Check sheet for the modelled part. Datum: model origin and axes. Units: mm. Coordinates: 2 decimals unless noted, no trailing zeros. Order: outer loops, then holes, each group sorted by start corner. A loop starts at its lowest first (then second) coordinate and runs counter-clockwise, first axis right, second up.
1. Cross-section at D-D (y = -14.5). Enter the section's corners in (x, z).
2. Draft check along Y on faces 1 (the cylindrical face through (4.68, 3.73, 0.99)), 2 (the flat face through (-20, -25.247, 1)), 3 (the flat face through (-11, -11, 0)). Enter one of: released by +Y, released by -Y, zero draft, split by the parting line, or undercut.
3. Cross-section at A-A (x = 0). Enter the section's corners in (y, z).
4. Cross-section at C-C (z = 1.3). Count the separate pieces of the cut face and the enclosed holes in it, then the cut area to 3 significant figures.
5. Cross-section at B-B (y = -7). Enter the section's corners in (x, z).
6. Thickness scan on line 1 (Y direction, x = 0, z = 0.6); line 2 (X direction, y = -5, z = 0.3); line 3 (X direction, y = -4, z = 1.9). Record the ranges inside material, lowest first.
7. Gauge pin test, flat ends, axial feed: pin 1 Ø2 at (x, y) = (7, 0) entering from -Z; pin 2 Ø2 at (x, y) = (-10, -9) entering from -Z; pin 3 Ø1 at (x, z) = (-35, 0.5) entering from +Y; pin 4 Ø1 at (y, z) = (-17, 1) entering from +X. Record the tip position at first contact, or that the pin passes through.
```python
from build123d import *

# Parameters (mm, degrees)
SKETCH_1_R      = 3
SKETCH_1_R_2    = 1.25
SKETCH_1_R_3    = 1
EXTRUDE_1_DEPTH = 2


with BuildPart() as part:
    # 草圖1 → 填料-伸長1 (new body)
    with BuildSketch(Plane.XY):
        with BuildLine():
            Line((-41.078680873, -25.246867961), (3.125001345, -25.246867961))
            Line((3.125001345, -25.246867961), (4.000056753, -25.246867961))
            Line((4.000056753, -25.246867961), (9.701825934, -2.423751958))
            ThreePointArc((9.701825934, -2.423751958), (5.1603748, 8.56566004), (-6.677431122, 7.443917894))
            Line((-6.677431122, 7.443917894), (-43.120716176, -25.246867961))
            Line((-43.120716176, -25.246867961), (-41.078680873, -25.246867961))
        make_face()
        Circle(SKETCH_1_R, mode=Mode.SUBTRACT)
        with Locations((0, 7)):
            Circle(SKETCH_1_R_2, mode=Mode.SUBTRACT)
        with Locations((4.949747468, 4.949747468)):
            Circle(SKETCH_1_R_2, mode=Mode.SUBTRACT)
        with Locations((7, 0)):
            Circle(SKETCH_1_R_2, mode=Mode.SUBTRACT)
        with Locations((4.949747468, -4.949747468)):
            Circle(SKETCH_1_R_2, mode=Mode.SUBTRACT)
        with Locations((0, -7)):
            Circle(SKETCH_1_R_2, mode=Mode.SUBTRACT)
        with Locations((-4.949747468, -4.949747468)):
            Circle(SKETCH_1_R_2, mode=Mode.SUBTRACT)
        with Locations((-7, 0)):
            Circle(SKETCH_1_R_2, mode=Mode.SUBTRACT)
        with Locations((-4.949747468, 4.949747468)):
            Circle(SKETCH_1_R_2, mode=Mode.SUBTRACT)
        with Locations((-13.732609449, -23.246867961)):
            Circle(SKETCH_1_R_3, mode=Mode.SUBTRACT)
        with Locations((-25.732609449, -23.246867961)):
            Circle(SKETCH_1_R_3, mode=Mode.SUBTRACT)
    extrude(amount=EXTRUDE_1_DEPTH)


solid = part.part
```
Data:
1. outline: (-31.14, 0) - (6.68, 0) - (6.68, 2) - (-31.14, 2) - close
2. face 1: undercut
2. face 2: released by -Y
2. face 3: zero draft
3. outline: (-25.25, 0) - (-8.25, 0) - (-8.25, 2) - (-25.25, 2) - close; (-5.75, 0) - (-3, 0) - (-3, 2) - (-5.75, 2) - close; (3, 0) - (5.75, 0) - (5.75, 2) - (3, 2) - close; (8.25, 0) - (10, 0) - (10, 2) - (8.25, 2) - close
4. separate pieces: 1
4. enclosed holes: 11
4. area: 1,010 mm2
5. outline: (-22.78, 0) - (-1.25, 0) - (-1.25, 2) - (-22.78, 2) - close; (1.25, 0) - (8.56, 0) - (8.56, 2) - (1.25, 2) - close
6. line 1: y = -25.25 to -8.25, -5.75 to -3, 3 to 5.75, 8.25 to 10
6. line 2: x = -20.55 to -6.2, -3.7 to 3.7, 6.2 to 9.06
6. line 3: x = -19.43 to -5.76, -4.14 to 4.14, 5.76 to 9.31
7. pin 1: passes through
7. pin 2: stops at z = 0
7. pin 3: stops at y = -17.51
7. pin 4: stops at x = 6.19
